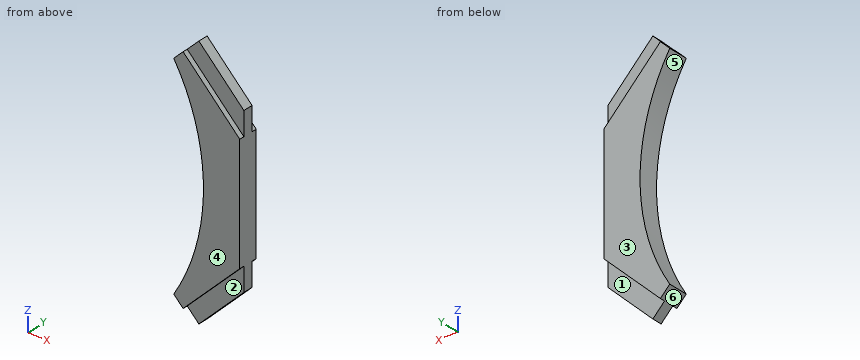
```python
from build123d import *

# Parameters (mm, degrees)
F1_DEPTH = 38.1
F2_DEPTH = 19.05


with BuildPart() as f1:
    # F0 (on Front) → F1 (new body, symmetric)
    with BuildSketch(Plane.XZ):
        with BuildLine():
            Line((127, 289.350815773), (-127, 543.350815773))
            ThreePointArc((-127, 543.350815773), (-12.7, 139.2408841362), (-127, -264.8690475006))
            Line((-127, -264.8690475006), (127, -10.8690475006))
            Line((127, -10.8690475006), (127, 289.350815773))
        make_face()
        Polygon((127, -10.8690475006), (-127, -264.8690475006), (-100.0592316368, -291.8098158638), (127, -64.750584227), align=None)
        Polygon((-100.0592316368, 570.2915841362), (-127, 543.350815773), (127, 289.350815773), (127, 343.2323524994), align=None)
        Polygon((-91.0789755157, 579.2718402573), (-100.0592316368, 570.2915841362), (127, 343.2323524994), (127, 361.1928647416), align=None)
        Polygon((127, -64.750584227), (-100.0592316368, -291.8098158638), (-91.0789755157, -300.7900719849), (127, -82.7110964691), align=None)
    extrude(amount=F1_DEPTH, both=True)

    # F0 (on Front) → F2 (join, symmetric)
    with BuildSketch(Plane.XZ):
        Polygon((127, 361.1928647416), (127, 450.9954259523), (-46.1776949104, 624.1731208626), (-91.0789755157, 579.2718402573), align=None)
        Polygon((127, -82.7110964691), (-91.0789755157, -300.7900719849), (-46.1776949104, -345.6913525902), (127, -172.5136576798), align=None)
    extrude(amount=F2_DEPTH, both=True)


solid = f1.part
```
Here's how the part is built. I have some questions about the finished solid (model axes, mm). Face numbers are marked on the shaded views. A direction names the side the tool comes from. Coordinates: 2 decimals unless noted, no trailing zeros. Order: outer loops, then holes, each group sorted by start corner. A loop starts at its lowest first (then second) coordinate and runs counter-clockwise, first axis right, second up. Notation, with made-up numbers: M -6,79.25 L 27,79.25 A6 ccw 27,89.25 Z; hole C 24,-26 d4. An arc over 180 degrees is marked long. Answer as a JSON object with one key per item and string values. Group by question number.
(1) Suppose I cut it at C-C, the plane y = -8. Please give me the cut outline in (x, z), then the cut area to 3 significant figures.
(2) If we mould it in two halves opening along Z, with no side actions, what happens to the marked faces 4, 5 and 6? For each: released by +Z, released by -Z, zero draft, split by the parting line, or undercut.
(3) Suppose I cut it at D-D, the plane x = 45.5. Please give me the cut outline in (y, z).
(4) Which directions (+Z, -Z, +X, -X, +Y, -Y) give clear straight access to the entire face, cutting with the end or side of a thin tool? Please do the marked faces 1, 2 and 3.
(5) I need wall thicknesses on probe 1 along Z at (x, y) = (-87, -1); probe 2 along Y at (x, z) = (73, -161); probe 3 along Z at (x, y) = (2.5, 9). Which ranges of each line are inside material? Lowest first, please.
(6) Suppose I cut it at A-A, the plane x = -108.5. Please give me the cut outline in (y, z).
(7) Suppose I cut it at B-B, the plane z = -285. Please give me the cut outline in (x, y).
(8) For pin 1 (1.5 mm diameter, centred on x = 58.5, y = -6, fed in from +Z); pin 2 (1 mm diameter, centred on x = 9.5, y = 25, fed in from -Z); pin 3 (8 mm diameter, centred on x = 92.5, y = 22.5, fed in from -Z), each with a flat end and sliding along its axis, tell me the tip position at first contact or that it passes through.
Values found:
{
 "1": {"outline": "M -127,-264.87 L -46.18,-345.69 L 127,-172.51 L 127,451 L -46.18,624.17 L -127,543.35 A771.52 cw Z", "area": "147,000 mm^2"},
 "2": {"face 4": "zero draft", "face 5": "undercut", "face 6": "released by -Z"},
 "3": {"outline": "M -38.1,-164.21 L -19.05,-164.21 L -19.05,-254.01 L 19.05,-254.01 L 19.05,-164.21 L 38.1,-164.21 L 38.1,442.69 L 19.05,442.69 L 19.05,532.5 L -19.05,532.5 L -19.05,442.69 L -38.1,442.69 Z"},
 "4": {"face 1": "-Z, +X, +Y", "face 2": "-Z, +X, -Y", "face 3": "+Z, -Z, +X, -X, +Y"},
 "5": {"probe 1": "z = -304.87 to -191.1, 469.59 to 583.35", "probe 2": "y = -19.05 to 19.05", "probe 3": "z = -297.01 to 575.5"},
 "6": {"outline": "M -38.1,-283.37 L 38.1,-283.37 L 38.1,-233.11 L -38.1,-233.11 Z; M -38.1,511.59 L 38.1,511.59 L 38.1,561.85 L -38.1,561.85 Z"},
 "7": {"outline": "M -106.87,-38.1 L -75.29,-38.1 L -75.29,-19.05 L 14.51,-19.05 L 14.51,19.05 L -75.29,19.05 L -75.29,38.1 L -106.87,38.1 Z"},
 "8": {"pin 1": "stops at z = 520.25", "pin 2": "stops at z = -200.71", "pin 3": "stops at z = -209.04"}
}
